```python
from build123d import *

# Parameters (mm, degrees)
F0_R      = 3.48
F1_DEPTH  = 6.88
F2_R      = 1.12
F3_DEPTH  = 6.23
F5_DEPTH  = 25
F7_DEPTH  = 6.88
F8_W      = 5.37
F8_H      = 4.36
F9_DEPTH  = 2.32
F10_R     = 2.4
F11_DEPTH = 1.93
F12_R     = 2.42
F13_DEPTH = 4.99


# Not quite as in the source:
# - a feature names something its author has since deleted; it is built from what else it names


with BuildPart() as f1:
    # F0 (on Front) → F1 (new body)
    with BuildSketch(Plane.XZ):
        Circle(F0_R)
    extrude(amount=F1_DEPTH)

    # F2 (on face) → F3 (cut)
    with BuildSketch(Plane.XZ.offset(6.88)):
        Circle(F2_R)
    extrude(amount=-F3_DEPTH, mode=Mode.SUBTRACT)

    # F4 (on face) → F5 (cut)
    with BuildSketch(Plane.XZ.offset(6.88)):
        Polygon((7.0880088024, -1.4447768917), (3.33, 4.3651785166), (3.33, -5.8573421486), align=None)
    extrude(amount=-F5_DEPTH, mode=Mode.SUBTRACT)

    # F6 (on face) → F7 (join)
    with BuildSketch(Plane.XZ.offset(6.88)):
        with BuildLine():
            Line((3.33, -10.3206928317), (3.33, -1.0106928317))
            ThreePointArc((3.33, -1.0106928317), (0.8809060484, -2.9691576427), (-2.24, -2.6632311203))
            Line((-2.24, -2.6632311203), (-2.24, -6.9906928317))
            Line((-2.24, -6.9906928317), (-4.56, -6.9906928317))
            Line((-4.56, -6.9906928317), (-4.56, -10.3206928317))
            Line((-4.56, -10.3206928317), (3.33, -10.3206928317))
        make_face()
    extrude(amount=-F7_DEPTH)

    # F8 (on face) → F9 (cut)
    with BuildSketch(Plane(origin=(0, 0, -10.3206928317), x_dir=(1, 0, 0), z_dir=(0, 0, -1))):
        with Locations((-0.615, 3.44)):
            Rectangle(F8_W, F8_H)
    extrude(amount=-F9_DEPTH, mode=Mode.SUBTRACT)

    # F10 (on face) → F11 (cut)
    with BuildSketch(Plane.YZ.offset(3.33)):
        with Locations((-3.44, 0)):
            Circle(F10_R)
    extrude(amount=-F11_DEPTH, mode=Mode.SUBTRACT)

    # F12 (on face) → F13 (cut)
    with BuildSketch(Plane.YZ.offset(3.33)):
        with Locations((-3.44, -6.2506928317)):
            Circle(F12_R)
    extrude(amount=-F13_DEPTH, mode=Mode.SUBTRACT)


solid = f1.part
```
Check sheet for the modelled part. Datum: model origin and axes. Units: mm. A direction names the side the tool comes from. Give positions to 0.01 mm unless a question says otherwise; leave off trailing zeros. Write each loop counter-clockwise with the first axis right and the second up, starting at its lowest first coordinate (ties: lowest second). Pieces come first, ordered by that corner, then holes.
Item 1: Cross-section at C-C (y = -6). Enter the section's corners in (x, z), and give its area (3 significant figures).
Item 2: Cross-section at A-A (y = -3.44). Enter the section's corners in (x, z).
Item 3: Cross-section at B-B (z = 0). Enter the section's corners in (x, y), and give its area (3 significant figures).
Item 4: Access from +Z, -Z, +X, -X, +Y, -Y to the whole of each face (thin tool, end or side, straight path). Record for faces 4 (the face through (-0.89, -3.81, -0.68)), 5 (the face through (-2.24, -3, -5)), 6 (the face through (-1, -5.62, -9)), 7 (the face through (0.87, -3.76, -3.85)).
Item 5: Cross-section at D-D (x = -1.5). Enter the section's corners in (y, z), and give its area (3 significant figures).
Item 6: Gauge pin test, flat ends, axial feed: pin 1 (3 mm diameter, centred on x = -2.5, z = -6, fed in from +Y); pin 2 (0.7 mm diameter, centred on x = -4, y = -2.5, fed in from +Z); pin 3 (0.7 mm diameter, centred on x = 0, z = -0.5, fed in from -Y); pin 4 (1.4 mm diameter, centred on y = -3, z = 0.5, fed in from +X). Record the tip position at first contact, or that the pin passes through.
Item 7: Scan lines: L1, parallel to Z at x = 2.1, y = -3.44; L2, parallel to Z at x = 2.25, y = -3.44; L3, parallel to Z at x = 2.9, y = -3.44. Record each from-to range of solid material in increasing order.
Item 8: Draft check along Y on faces 1 (the face through (0, -0.65, 0)), 2 (the face through (-3.3, -3, -9)), 3 (the face through (0, 0, -3)). Enter one of: released by +Y, released by -Y, zero draft, split by the parting line, or undercut.
Report:
1. outline: (-4.56, -10.32) - (3.33, -10.32) - (3.33, 1.01) arc R3.48 ccw (long way) to (-2.24, -2.66) - (-2.24, -6.99) - (-4.56, -6.99) - close; hole circle Ø2.24 at (0, 0)
1. area: 82.5 mm2
2. outline: (-4.56, -10.32) - (-3.3, -10.32) - (-3.3, -8) - (-1.66, -8) - (-1.66, -3.83) - (3.33, -3.83) - (3.33, -2.4) - (1.4, -2.4) - (1.4, 2.4) - (2.52, 2.4) arc R3.48 ccw (long way) to (-2.24, -2.66) - (-2.24, -6.99) - (-4.56, -6.99) - close; (2.07, -10.32) - (3.33, -10.32) - (3.33, -8.67) - (2.07, -8.67) - close; hole circle Ø2.24 at (0, 0)
3. outline: (-3.48, -6.88) - (-1.12, -6.88) - (-1.12, -0.65) - (1.12, -0.65) - (1.12, -6.88) - (3.33, -6.88) - (3.33, -5.84) - (1.4, -5.84) - (1.4, -1.04) - (3.33, -1.04) - (3.33, 0) - (-3.48, 0) - close
3. area: 23.6 mm2
4. face 4: -Y
4. face 5: -X, +Y, -Y
4. face 6: -Z
4. face 7: +X
5. outline: (-6.88, -10.32) - (-5.62, -10.32) - (-5.62, -8) - (-5.11, -8) arc R2.42 cw (long way) to (-1.77, -8) - (-1.26, -8) - (-1.26, -10.32) - (0, -10.32) - (0, 3.14) - (-6.88, 3.14) - close
5. area: 65.6 mm2
6. pin 1: stops at y = 0
6. pin 2: stops at z = -6.99
6. pin 3: stops at y = -0.65
6. pin 4: stops at x = 1.4
7. L1: z = -10.32 to -8.67, -3.83 to -2.4, 2.4 to 2.77
7. L2: z = -10.32 to -8.67, -3.83 to -2.4, 2.4 to 2.65
7. L3: z = -10.32 to -8.67, -3.83 to -2.4
8. face 1: released by -Y
8. face 2: undercut
8. face 3: released by +Y
